Autodesk Inventor part; units mm, degrees
ref_plane "YZ Plane" through (0, 0, 0) normal (1, 0, 0) x (0, 1, 0)
ref_plane "XZ Plane" through (0, 0, 0) normal (0, 1, 0) x (-1, 0, 0)
ref_plane "XY Plane" through (0, 0, 0) normal (0, 0, 1) x (1, 0, 0)
sketch "Sketch1" plane through (0, 0, 0) normal (0, 0, 1) x (1, 0, 0)
  ellipse E0 centre (0, 0) end of major axis (0, 3.5) minor radius 3.5
  arc A0 (-2.0076, 1.85) -> (-2.0076, -1.85) centre (0, 0) ccw
  line L0 (-2.0076, 1.85) -> (2.0076, 1.85)
  arc A1 (2.0076, -1.85) -> (2.0076, 1.85) centre (0, 0) ccw
  line L1 (2.0076, -1.85) -> (-2.0076, -1.85)
  line L2 (-50, -25) -> (50, -25)
  line L3 (50, -25) -> (50, 25)
  line L4 (50, 25) -> (-50, 25)
  line L5 (-50, 25) -> (-50, -25)
  line L6 (-50, -25) -> (50, 25) construction
  line L7 (50, -25) -> (-50, 25) construction
  line L8 (-25, -25) -> (-25, 25)
  line L9 (25, -25) -> (25, 25)
  circle A2 centre (0, 0) radius 6.15
  point P0 (0, 0)
  dimension "d0" = 100
  dimension "d1" = 50
  dimension "d4" = 25
  dimension "d5" = 50
  dimension "d10" = 12.3
extrude "Extrusion1" add sketch "Sketch1" against normal blind 3 contours L8 L4 L9 L2
sketch "Sketch2" plane through (0, 0, -3) normal (0, 0, -1) x (-1, 0, 0)
  circle A0 centre (20.11, -8.75) radius 1.5
  circle A1 centre (11.22, 0) radius 2.08
  circle A2 centre (20.11, 8.75) radius 1.5
  point P0 (0, 0)
extrude "Extrusion2" cut sketch "Sketch2" against normal through all
sketch "Sketch3" plane through (-25, -25, 0) normal (-1, 0, 0) x (0, 0, 1)
  line L0 (0, 50) -> (0, 0)
  line L1 (0, 50) -> (-3, 50)
  line L2 (-3, 0) -> (-3, 50)
  line L3 (0, 0) -> (-3, 0)
  point P0 (0, 25)
extrude "Extrusion3" add sketch "Sketch3" along normal blind 10
sketch "Sketch4" plane through (0, 0, -3) normal (0, 0, -1) x (-1, 0, 0)
  circle A0 centre (20.11, -8.75) radius 1.5
  circle A1 centre (20.11, 8.75) radius 1.5
  point P0 (0, 0)
extrude "Extrusion4" cut sketch "Sketch4" against normal through all
properties part number "arm2"
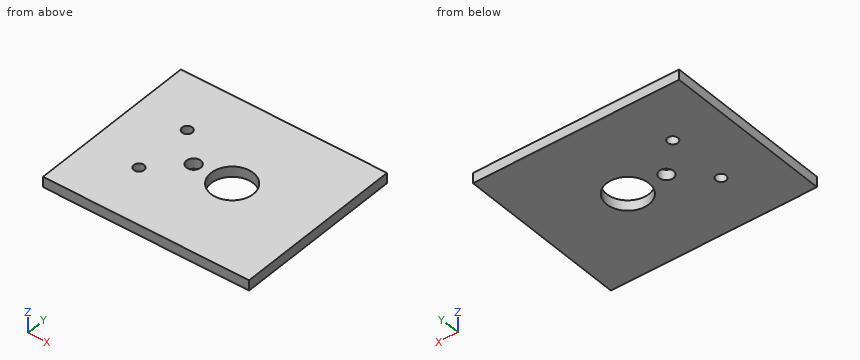
The listing builds one solid part. Answer for the finished solid, in the listing's coordinates (mm). Give positions to 0.01 mm unless a question says otherwise; leave off trailing zeros. Loops run counter-clockwise (first coordinate to the right, second up) from the corner with the lowest first, then second, coordinate; pieces in that order, holes last. Notation, with made-up numbers: (5, 77.25) - (22, 77.25) arc R12 cw to (22, 97.25) - close; hole circle Ø1 at (43, -12.5). An arc over 180 degrees is marked (long way). Return JSON: item names as keys, results as strings. Group by question number.
1. Straight lines are drawn through the part: line 1 (Y direction, x = -11.22, z = -1); line 2 (Y direction, x = -20.11, z = -1.5); line 3 (Y direction, x = 0, z = -2.3). For each, find the intervals that lie inside material, in ascending order. Write a range as [from, to].
2. Find section A-A (y = -8.75). Write down the section's boundary in (x, z).
3. Find section D-D (y = 0). Write down the section's boundary in (x, z), then the cut area to 3 significant figures.
4. Find section C-C (x = 0). Write down the section's boundary in (y, z).
5. Find section B-B (x = -20.11). Write down the section's boundary in (y, z), then the cut area to 3 significant figures.
Verdict:
{
 "1": {"line 1": "y = [-25, -2.08], [2.08, 25]", "line 2": "y = [-25, -10.25], [-7.25, 7.25], [10.25, 25]", "line 3": "y = [-25, -6.15], [6.15, 25]"},
 "2": {"outline": "(-35, -3) - (-21.61, -3) - (-21.61, 0) - (-35, 0) - close; (-18.61, -3) - (25, -3) - (25, 0) - (-18.61, 0) - close"},
 "3": {"outline": "(-35, -3) - (-13.3, -3) - (-13.3, 0) - (-35, 0) - close; (-9.14, -3) - (-6.15, -3) - (-6.15, 0) - (-9.14, 0) - close; (6.15, -3) - (25, -3) - (25, 0) - (6.15, 0) - close", "area": "131 mm^2"},
 "4": {"outline": "(-25, -3) - (-6.15, -3) - (-6.15, 0) - (-25, 0) - close; (6.15, -3) - (25, -3) - (25, 0) - (6.15, 0) - close"},
 "5": {"outline": "(-25, -3) - (-10.25, -3) - (-10.25, 0) - (-25, 0) - close; (-7.25, -3) - (7.25, -3) - (7.25, 0) - (-7.25, 0) - close; (10.25, -3) - (25, -3) - (25, 0) - (10.25, 0) - close", "area": "132 mm^2"}
}
